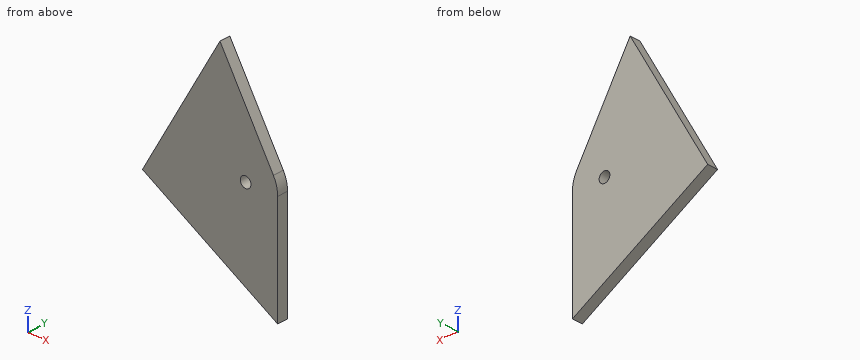
from build123d import *

# Parameters (mm, degrees)
ESQUISSE1_R        = 1
BOSS_EXTRU_1_DEPTH = 2


with BuildPart() as part:
    # Esquisse1 → Boss.-Extru.1 (new body)
    with BuildSketch(Plane(origin=(0, 0, 0), x_dir=(1, 0, 0), z_dir=(0, 1, 0))):
        with BuildLine():
            Line((6, 0), (6, 20))
            Line((6, 20), (-19.318516526, 5.176380902))
            Line((-19.318516526, 5.176380902), (-4.803847577, -20.320508076))
            Line((-4.803847577, -20.320508076), (5.196152423, -3))
            ThreePointArc((5.196152423, -3), (5.795554958, -1.552914271), (6, 0))
        make_face()
        Circle(ESQUISSE1_R, mode=Mode.SUBTRACT)
    extrude(amount=BOSS_EXTRU_1_DEPTH)


solid = part.part
Design review of the part built by this model. Coordinates are the model's own, in mm. Round coordinates to 2 decimals unless told otherwise and drop trailing zeros. Write each loop counter-clockwise with the first axis right and the second up, starting at its lowest first coordinate (ties: lowest second). Pieces come first, ordered by that corner, then holes. Notation, with made-up numbers: (29, 73) -> (54, 73) arc R29 cw to (54, 103) -> close; hole circle Ø4 at (16.5, -37). An arc over 180 degrees is marked (long way). One line per item, written item: value. Start each with the question number.
Q1. Add section D-D (x = 2.75). Give the boundary of the cut face in (y, z).
Q2. Insertion check: P1, Ø2, axis at x = 3, z = -15.5, coming from the -Y side; P2, Ø1.8, axis at x = 0, z = 0, coming from the -Y side. Each pin has a flat end and moves straight along its axis. Give the tip position at first contact, or say it passes through.
Q3. Add section A-A (x = 0). Give the boundary of the cut face in (y, z).
Q4. Add section C-C (z = 16.5). Give the boundary of the cut face in (x, y), then the cut area to 3 significant figures.
Q5. Add section B-B (y = 1.1). Give the boundary of the cut face in (x, z).
Q6. To check wall thickness, follow probe 1 along Z at (x, y) = (0, 0.5); probe 2 along X at (y, z) = (0.95, 6); probe 3 along X at (y, z) = (1.4, -14). State the ranges of each line that lie inside material, in increasing order.
Response:
1. outline: (0, -18.1) -> (2, -18.1) -> (2, 7.24) -> (0, 7.24) -> close
2. P1: stops at y = 0
2. P2: passes through
3. outline: (0, -16.49) -> (2, -16.49) -> (2, -1) -> (0, -1) -> close; (0, 1) -> (2, 1) -> (2, 12) -> (0, 12) -> close
4. outline: (-6.98, 0) -> (-2.6, 0) -> (-2.6, 2) -> (-6.98, 2) -> close
4. area: 8.76 mm^2
5. outline: (-19.32, -5.18) -> (6, -20) -> (6, 0) arc R6 ccw to (5.2, 3) -> (-4.8, 20.32) -> close; hole circle Ø2 at (0, 0)
6. probe 1: z = -16.49 to -1, 1 to 12
6. probe 2: x = -12.96 to 3.46
6. probe 3: x = -4.25 to 6
